Geometry check sheet. Reference: drawing and pictorial views, mm from the part's lowest x, y, z. Round coordinates to 2 decimals unless told otherwise and drop trailing zeros. Loops run counter-clockwise (first coordinate to the right, second up) from the corner with the lowest first, then second, coordinate; pieces in that order, holes last. Notation, with made-up numbers: M -9,21 L 49,21 A16 ccw 49,33 Z; hole C -28.5,82.25 d7. An arc over 180 degrees is marked long. One line per question, with ' | ' between items. Start each with the question number.
(1) Go/stop test with flat-tipped pins: P1, Ø6, axis at x = 12, y = 10, coming from the +Z side; P2, Ø1, axis at y = 51, z = 2, coming from the -X side. Record where each tip stops, or that it passes through.
(2) Section check C-C (z = 2.3). Record the boundary of the cut face in (x, y), and give its area (3 significant figures).
(3) Thickness scan on probe 1 along Y at (x, z) = (25, 2.4); probe 2 along Y at (x, z) = (12, 3.85); probe 3 along Y at (x, z) = (7, 3.2). Record the ranges inside material, lowest first. Write a range as [from, to].
(4) Section check A-A (x = 25). Record the boundary of the cut face in (y, z), and give its area (3 significant figures).
(5) Draft check along X on the marked faces 1, 2 and 3. Enter one of: +X half, -X half, draft (parallel to the pull), parting line (faces both ways), or undercut.
(6) Section check B-B (y = 10). Record the boundary of the cut face in (x, z).
(7) Section check D-D (x = 9.5). Record the boundary of the cut face in (y, z), and give its area (3 significant figures).
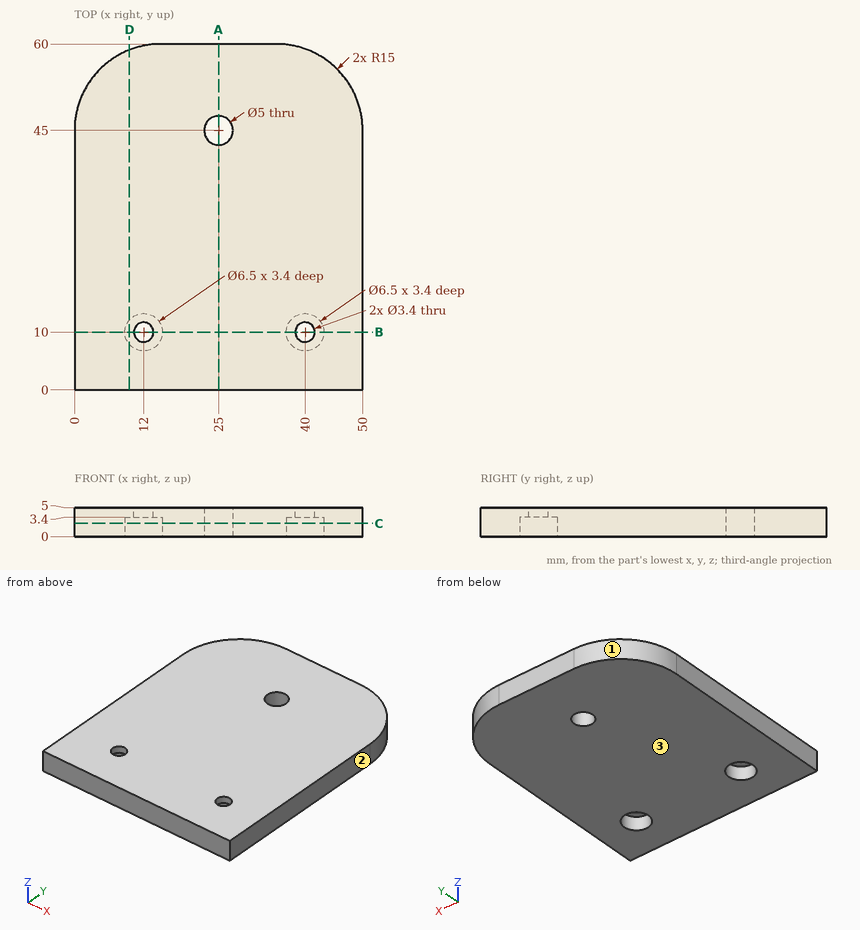
The answers:
1) P1: z = 5 | P2: x = 1.04
2) outline: M 0,0 L 50,0 L 50,45 A15 ccw 35,60 L 15,60 A15 ccw 0,45 Z; hole C 12,10 d6.5; hole C 25,45 d5; hole C 40,10 d6.5 | area: 2,820 mm²
3) probe 1: [0, 42.5], [47.5, 60] | probe 2: [0, 8.3], [11.7, 59.7] | probe 3: [0, 57.69]
4) outline: M 0,0 L 42.5,0 L 42.5,5 L 0,5 Z; M 47.5,0 L 60,0 L 60,5 L 47.5,5 Z | area: 275 mm²
5) face 1: -X half | face 2: +X half | face 3: draft
6) outline: M 0,0 L 8.75,0 L 8.75,3.4 L 10.3,3.4 L 10.3,5 L 0,5 Z; M 13.7,3.4 L 15.25,3.4 L 15.25,0 L 36.75,0 L 36.75,3.4 L 38.3,3.4 L 38.3,5 L 13.7,5 Z; M 41.7,3.4 L 43.25,3.4 L 43.25,0 L 50,0 L 50,5 L 41.7,5 Z
7) outline: M 0,0 L 7.92,0 L 7.92,3.4 L 12.08,3.4 L 12.08,0 L 58.96,0 L 58.96,5 L 0,5 Z | area: 281 mm²
